Input: part model. Units: mm. Frame: model coordinates. Give positions to 0.01 mm unless a question says otherwise; leave off trailing zeros. Write each loop counter-clockwise with the first axis right and the second up, starting at its lowest first coordinate (ties: lowest second). Pieces come first, ordered by that corner, then holes. Notation, with made-up numbers: (38, 16) -> (46, 16) arc R16 cw to (46, 27) -> close; hole circle Ø3 at (-19, 3). An arc over 180 degrees is marked (long way). Return JSON: item names as keys, results as strings. Group by question number.
Item 1: Section D-D, the plane x = 16. Return loops of the section in (y, z) (3 decimals).
Item 2: Mould query, pull axis X, two halves, no side actions, for faces 1 (the face through (14.274, 0.628, 9.392)), 2 (the face through (-2.75, -12.4, 11.27)), 3 (the face through (-2.7, 14.2, 19.05)). Classes: released by +X, released by -X, zero draft, split by the parting line, or undercut.
Item 3: Line query: line 1 (Y direction, x = 0, z = 17.75); line 2 (Y direction, x = -3.5, z = 6); line 3 (Z direction, x = 16, y = 8.5) (3 decimals). Output: solid intervals per line, ascending. Write a range as [from, to].
Item 4: Pin query (flat end, axial travel): P1, Ø6, axis at y = -3.5, z = 2.5, coming from the +X side; P2, Ø10, axis at y = -1.5, z = 7.5, coming from the -X side; P3, Ø1, axis at y = 8.5, z = 9.5, coming from the -X side. Return the tip coordinate at first contact, or that it passes through.
Item 5: Section C-C, the plane z = 4. Return loops of the section in (x, y) (1 decimal), then the cut area to 3 significant figures.
from build123d import *

# Parameters (mm, degrees)
SKETCH1_R           = 19.05
BOSS_EXTRUDE1_DEPTH = 22.225
SKETCH2_R           = 19.05
SKETCH2_R_2         = 14.2875
CUT_EXTRUDE1_DEPTH  = 19.05
SKETCH3_R           = 12.7
CUT_EXTRUDE2_DEPTH  = 35.925


with BuildPart() as part:
    # Sketch1 → Boss-Extrude1 (new body)
    with BuildSketch(Plane.XY):
        Circle(SKETCH1_R)
    extrude(amount=BOSS_EXTRUDE1_DEPTH)

    # Sketch2 → Cut-Extrude1 (cut)
    with BuildSketch(Plane(origin=(0, 0, 0), x_dir=(-1, 0, 0), z_dir=(0, 0, -1))):
        Circle(SKETCH2_R)
        Circle(SKETCH2_R_2, mode=Mode.SUBTRACT)
    extrude(amount=-CUT_EXTRUDE1_DEPTH, mode=Mode.SUBTRACT)

    # Sketch3 → Cut-Extrude2 (cut, through all)
    with BuildSketch(Plane.XY.offset(22.225)):
        Circle(SKETCH3_R)
    extrude(amount=-CUT_EXTRUDE2_DEPTH, mode=Mode.SUBTRACT)


solid = part.part
Answer below:
{
 "1": {"outline": "(-10.339, 19.05) -> (10.339, 19.05) -> (10.339, 22.225) -> (-10.339, 22.225) -> close"},
 "2": {"face 1": "split by the parting line", "face 2": "undercut", "face 3": "zero draft"},
 "3": {"line 1": "y = [-14.29, -12.7], [12.7, 14.29]", "line 2": "y = [-13.85, -12.21], [12.21, 13.85]", "line 3": "z = [19.05, 22.225]"},
 "4": {"P1": "stops at x = 14.28", "P2": "stops at x = -14.29", "P3": "stops at x = -11.84"},
 "5": {"outline": "circle Ø28.6 at (0, 0); hole circle Ø25.4 at (0, 0)", "area": "135 mm2"}
}
